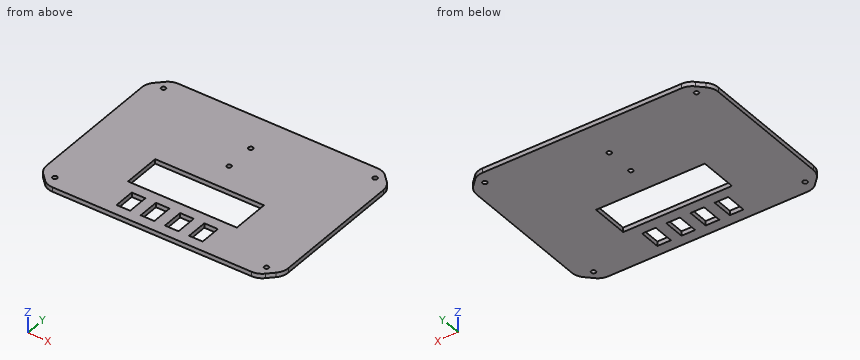
```python
from build123d import *

# Parameters (mm, degrees)
BOSS_EXTRUDE1_DEPTH     = 3
CUT_EXTRUDE1_DEPTH      = 141.943250991
CUT_EXTRUDE1_DEPTH_BACK = 3
CUT_EXTRUDE2_DEPTH      = 141.943250991
CUT_EXTRUDE2_DEPTH_BACK = 3
SKETCH5_R               = 1.5
SKETCH5_W               = 72
SKETCH5_H               = 25
SKETCH5_W_2             = 9
SKETCH5_H_2             = 14
CUT_EXTRUDE3_DEPTH      = 141.943250991
FILLET1_R               = 10


with BuildPart() as part:
    # Sketch1 → Boss-Extrude1 (new body)
    with BuildSketch(Plane.XY):
        Polygon((80, 116), (-80, 116), (-80, 10), (-70, 0), (70, 0), (80, 10), align=None)
    extrude(amount=BOSS_EXTRUDE1_DEPTH)

    # Sketch3 → Cut-Extrude1 (cut, two sides: drawn at the far end of the back side and taken through both)
    with BuildSketch(Plane(origin=(0, 0, 0), x_dir=(-1, 0, 0), z_dir=(0, 0, -1)).offset(-CUT_EXTRUDE1_DEPTH_BACK)):
        Polygon((-358.49693246, -172.49693246), (-80, 106), (-70, 116), (208.49693246, 394.49693246), (-348.49693246, 951.49079738), (-915.49079738, 384.49693246), align=None)
    extrude(amount=CUT_EXTRUDE1_DEPTH + CUT_EXTRUDE1_DEPTH_BACK, mode=Mode.SUBTRACT)

    # Sketch4 → Cut-Extrude2 (cut, two sides: drawn at the far end of the back side and taken through both)
    with BuildSketch(Plane(origin=(0, 0, 0), x_dir=(-1, 0, 0), z_dir=(0, 0, -1)).offset(-CUT_EXTRUDE2_DEPTH_BACK)):
        Polygon((-208.49693246, 394.49693246), (70, 116), (80, 106), (358.49693246, -172.49693246), (915.49079738, 384.49693246), (348.49693246, 951.49079738), align=None)
    extrude(amount=CUT_EXTRUDE2_DEPTH + CUT_EXTRUDE2_DEPTH_BACK, mode=Mode.SUBTRACT)

    # Sketch5 → Cut-Extrude3 (cut, through all)
    with BuildSketch(Plane(origin=(0, 0, 0), x_dir=(-1, 0, 0), z_dir=(0, 0, -1))):
        with Locations((0, 91)):
            Circle(SKETCH5_R)
        with Locations((0, 71)):
            Circle(SKETCH5_R)
        with Locations((-70, 8)):
            Circle(SKETCH5_R)
        with Locations((70, 8)):
            Circle(SKETCH5_R)
        with Locations((70, 108)):
            Circle(SKETCH5_R)
        with Locations((-70, 108)):
            Circle(SKETCH5_R)
        with Locations((0, 40.5)):
            Rectangle(SKETCH5_W, SKETCH5_H)
        with Locations((-24, 14)):
            Rectangle(SKETCH5_W_2, SKETCH5_H_2)
        with Locations((-8, 14)):
            Rectangle(SKETCH5_W_2, SKETCH5_H_2)
        with Locations((8, 14)):
            Rectangle(SKETCH5_W_2, SKETCH5_H_2)
        with Locations((24, 14)):
            Rectangle(SKETCH5_W_2, SKETCH5_H_2)
    extrude(amount=-CUT_EXTRUDE3_DEPTH, mode=Mode.SUBTRACT)

    # Fillet1
    fillet1_edges = [part.edges().sort_by_distance(p)[0] for p in [
        (-80, 10, 1.5),
        (80, 10, 1.5),
        (70, 0, 1.5),
        (-70, 0, 1.5),
        (80, 106, 1.5),
        (70, 116, 1.5),
        (-70, 116, 1.5),
        (-80, 106, 1.5),
    ]]
    fillet(fillet1_edges, radius=FILLET1_R)


solid = part.part
```
Check sheet for the modelled part. Datum: model origin and axes. Units: mm. Give positions to 0.01 mm unless a question says otherwise; leave off trailing zeros. Loops run counter-clockwise (first coordinate to the right, second up) from the corner with the lowest first, then second, coordinate; pieces in that order, holes last. Notation, with made-up numbers: (45, -17.75) - (59, -17.75) arc R28 ccw to (59, 15.25) - close; hole circle Ø8 at (-37, -10.75). An arc over 180 degrees is marked (long way). One line per question, with ' | ' between items. Start each with the question number.
1. Cross-section at A-A, the plane x = 34. Enter the section's corners in (y, z), plus the area to 3 significant figures.
2. Cross-section at C-C, the plane z = 1.2. Give the number of separate pieces and of enclosed holes in the cut face, plus the area to 3 significant figures.
3. Gauge pin test, flat ends, axial feed: pin 1 Ø4 at (x, y) = (29.5, 68) entering from -Z; pin 2 Ø0.9 at (y, z) = (10.5, 2) entering from +X; pin 3 Ø1.5 at (y, z) = (12.5, 1.5) entering from +X. Record the tip position at first contact, or that the pin passes through.
4. Cross-section at B-B, the plane y = 51. Enter the section's corners in (x, z).
5. Material ranges on line 1 along Y through (x, z) = (8.5, 1.1); line 2 along Y through (x, z) = (0, 1.75); line 3 along Y through (x, z) = (70, 0.8), recorded low to high. Write a range as [from, to].
Check result:
1) outline: (0, 0) - (28, 0) - (28, 3) - (0, 3) - close; (53, 0) - (116, 0) - (116, 3) - (53, 3) - close | area: 273 mm2
2) separate pieces: 1 | enclosed holes: 11 | area: 16,000 mm2
3) pin 1: stops at z = 0 | pin 2: stops at x = 79.48 | pin 3: stops at x = 79.96
4) outline: (-80, 0) - (-36, 0) - (-36, 3) - (-80, 3) - close; (36, 0) - (80, 0) - (80, 3) - (36, 3) - close
5) line 1: y = [0, 7], [21, 28], [53, 116] | line 2: y = [0, 28], [53, 69.5], [72.5, 89.5], [92.5, 116] | line 3: y = [0.9, 6.5], [9.5, 106.5], [109.5, 115.1]
